Here's how the part is built. I have some questions about the finished solid (model axes, mm). A direction names the side the tool comes from. Coordinates: 2 decimals unless noted, no trailing zeros. Write each loop counter-clockwise with the first axis right and the second up, starting at its lowest first coordinate (ties: lowest second). Pieces come first, ordered by that corner, then holes. Notation, with made-up numbers: (-14, 72) -> (0, 72) arc R6 ccw to (0, 77) -> close; hole circle Ø3 at (-35.5, -3.5). An arc over 180 degrees is marked (long way). Put each result on its own line as item: value.
```python
from build123d import *

# Parameters (mm, degrees)
F0_R     = 2.54
F1_DEPTH = 5.08
F2_W     = 63.5
F2_H     = 5.08
F3_DEPTH = 5.08
F5_DEPTH = 25.4


with BuildPart() as f1:
    # F0 (on Front) → F1 (new body)
    with BuildSketch(Plane.XZ):
        with BuildLine():
            Line((32.91078, 0), (0, 0))
            Line((0, 0), (0, -25.4))
            Line((0, -25.4), (18.62328, -25.4))
            ThreePointArc((18.62328, -25.4), (22.807992, -15.297212), (32.91078, -11.1125))
            Line((32.91078, -11.1125), (32.91078, 0))
        make_face()
        with BuildLine():
            Line((18.62328, -25.4), (0, -25.4))
            Line((0, -25.4), (0, -139.7))
            Line((0, -139.7), (139.7, -139.7))
            Line((139.7, -139.7), (187.900217, -139.7))
            Line((187.900217, -139.7), (187.900217, -109.5375))
            ThreePointArc((187.900217, -109.5375), (177.797429, -105.352788), (173.612717, -95.25))
            ThreePointArc((173.612717, -95.25), (173.931707, -92.247768), (174.874435, -89.379594))
            Line((174.874435, -89.379594), (45.936562, -31.270406))
            ThreePointArc((45.936562, -31.270406), (29.908548, -39.368509), (18.62328, -25.4))
        make_face()
        with Locations((162.900217, -95.25)):
            Circle(F0_R, mode=Mode.SUBTRACT)
        with BuildLine():
            Line((139.7, 0), (32.91078, 0))
            Line((32.91078, 0), (32.91078, -11.1125))
            ThreePointArc((32.91078, -11.1125), (43.013568, -15.297212), (47.19828, -25.4))
            ThreePointArc((47.19828, -25.4), (46.879289, -28.402232), (45.936562, -31.270406))
            Line((45.936562, -31.270406), (174.874435, -89.379594))
            ThreePointArc((174.874435, -89.379594), (190.902449, -81.281491), (202.187717, -95.25))
            ThreePointArc((202.187717, -95.25), (198.003005, -105.352788), (187.900217, -109.5375))
            Line((187.900217, -109.5375), (187.900217, -139.7))
            Line((187.900217, -139.7), (228.6, -139.7))
            Line((228.6, -139.7), (228.6, -38.1))
            Line((228.6, -38.1), (139.7, 0))
        make_face()
        with BuildLine():
            ThreePointArc((215.440217, -95.25), (212.900217, -97.79), (210.360217, -95.25))
            ThreePointArc((210.360217, -95.25), (212.900217, -92.71), (215.440217, -95.25))
        make_face(mode=Mode.SUBTRACT)
    extrude(amount=F1_DEPTH)

    # F2 (on face) → F3 (cut)
    with BuildSketch(Plane(origin=(0, 0, -139.7), x_dir=(1, 0, 0), z_dir=(0, 0, -1))):
        with Locations((69.85, 2.54)):
            Rectangle(F2_W, F2_H)
    extrude(amount=-F3_DEPTH, mode=Mode.SUBTRACT)

    # F4 (on face) → F5 (cut)
    with BuildSketch(Plane.XZ.offset(5.08)):
        Polygon((139.7, -69.85), (139.7, -101.6), (142.24, -101.6), (144.78, -101.6), (144.78, -38.1), (139.7, -38.1), align=None)
    extrude(amount=-F5_DEPTH, mode=Mode.SUBTRACT)


solid = f1.part
```
Item 1: Please list where these lines run through material, in increasing order: line 1 along X through (y, z) = (-0.75, -88); line 2 along X through (y, z) = (-2.15, -79.5); line 3 along Z through (x, y) = (197, -2.5). Write a range as from..to.
Output:
line 1: x = 0..139.7, 144.78..175.59, 200.21..228.6
line 2: x = 0..139.7, 144.78..228.6
line 3: z = -139.7..-106.26, -84.24..-24.56
Item 2: Imagine slicing it at C-C on x = 30.5. Write out the boundary of the cut face in (y, z).
Output:
outline: (-5.08, -139.7) -> (0, -139.7) -> (0, -39.48) -> (-5.08, -39.48) -> close; (-5.08, -11.32) -> (0, -11.32) -> (0, 0) -> (-5.08, 0) -> close
Item 3: Imagine slicing it at B-B on y = -2.5. State how many separate pieces and enclosed holes the cut face has, then the cut area to 3 significant figures.
Output:
separate pieces: 1
enclosed holes: 5
area: 28,300 mm²
Item 4: For P1, Ø1.5, axis at x = 71, y = -3, coming from the -Z side; P2, Ø2.5, axis at x = 141.5, y = -2, coming from the +Z side; P3, Ø2, axis at x = 204, y = -1.5, coming from the +Z side, each with a flat end and sliding along its axis, tell me the tip position at first contact or that it passes through.
Output:
P1: stops at z = -134.62
P2: stops at z = -0.24
P3: stops at z = -27.13
Item 5: Which directions (+Z, -Z, +X, -X, +Y, -Y) give clear straight access to the entire face, cutting with the end or side of a thin tool? Please do faces 1 (the flat face through (228.6, -3, -90)), 2 (the flat face through (142, -3, -38.1)), 3 (the flat face through (38.1, -3, -137)).
Output:
face 1: +Z, -Z, +X, +Y, -Y
face 2: +Y, -Y
face 3: -Z, +Y, -Y
Item 6: Imagine slicing it at A-A on z = -74. Write out the boundary of the cut face in (x, y), then the cut area to 3 significant figures.
Output:
outline: (0, -5.08) -> (139.7, -5.08) -> (139.7, 0) -> (0, 0) -> close; (144.78, -5.08) -> (228.6, -5.08) -> (228.6, 0) -> (144.78, 0) -> close
area: 1,140 mm²
Item 7: If we mould it in two halves opening along X, with no side actions, what happens to faces 4 (the flat face through (0, -3, -69)), 5 (the flat face through (164, -3, -139.7)), 6 (the flat face through (101.6, -3, -137))? For each: released by +X, released by -X, zero draft, split by the parting line, or undercut.
Output:
face 4: released by -X
face 5: zero draft
face 6: undercut
